Job drawing, mm, ordinate dimensions from the low corner. One solid piece. Round coordinates to 2 decimals unless told otherwise and drop trailing zeros. Order: outer loops, then holes, each group sorted by start corner. A loop starts at its lowest first (then second) coordinate and runs counter-clockwise, first axis right, second up. Notation, with made-up numbers: (15.25, 9.5) -> (57.25, 9.5) arc R20 ccw to (57.25, 48.5) -> close; hole circle Ø11 at (35, 71). An arc over 180 degrees is marked (long way). Use CSV: the item, a comma, the result in double quotes.
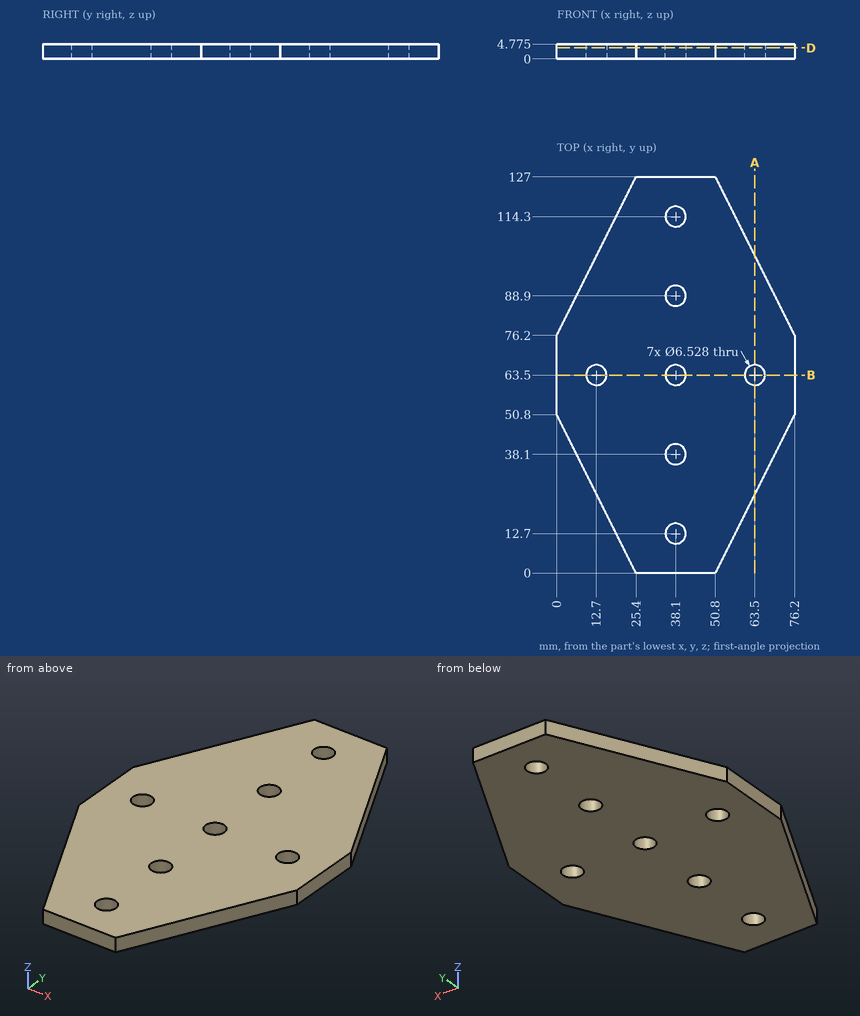
(1) Cut at B-B, the plane y = 63.5. Give the cut face in (x, z) (1 decimal).
Reply:
outline,"(0, 0) -> (9.4, 0) -> (9.4, 4.8) -> (0, 4.8) -> close; (16, 0) -> (34.8, 0) -> (34.8, 4.8) -> (16, 4.8) -> close; (41.4, 0) -> (60.2, 0) -> (60.2, 4.8) -> (41.4, 4.8) -> close; (66.8, 0) -> (76.2, 0) -> (76.2, 4.8) -> (66.8, 4.8) -> close"
(2) Probe probe 1 along Y at (x, z) = (38.1, 1.45); probe 2 along Y at (x, z) = (37.5, 0.6); probe 3 along Y at (x, z) = (63.5, 3.75) (1 decimal). List the from-to ranges inside material, lowest first. Write a range as [from, to].
Reply:
probe 1,"[0, 9.44], [15.96, 34.84], [41.36, 60.24], [66.76, 85.64], [92.16, 111.04], [117.56, 127]"
probe 2,"[0, 9.49], [15.91, 34.89], [41.31, 60.29], [66.71, 85.69], [92.11, 111.09], [117.51, 127]"
probe 3,"[25.4, 60.2], [66.8, 101.6]"
(3) Cut at D-D, the plane z = 3.5. Give the cut face in (x, y), then the cut area to 3 significant figures.
Reply:
outline,"(0, 50.8) -> (25.4, 0) -> (50.8, 0) -> (76.2, 50.8) -> (76.2, 76.2) -> (50.8, 127) -> (25.4, 127) -> (0, 76.2) -> close; hole circle Ø6.53 at (12.7, 63.5); hole circle Ø6.53 at (38.1, 12.7); hole circle Ø6.53 at (38.1, 38.1); hole circle Ø6.53 at (38.1, 63.5); hole circle Ø6.53 at (38.1, 88.9); hole circle Ø6.53 at (38.1, 114.3); hole circle Ø6.53 at (63.5, 63.5)"
area,"6,860 mm2"
(4) Cut at A-A, the plane x = 63.5. Give the cut face in (y, z) (1 decimal).
Reply:
outline,"(25.4, 0) -> (60.2, 0) -> (60.2, 4.8) -> (25.4, 4.8) -> close; (66.8, 0) -> (101.6, 0) -> (101.6, 4.8) -> (66.8, 4.8) -> close"
(5) Drop flat-ended pins along their axis: P1, Ø4, axis at x = 12.7, y = 63.5, coming from the -Z side; P2, Ø7.5, axis at x = 38.1, y = 114.3, coming from the +Z side (3 decimals); P3, Ø2, axis at y = 30, z = 1.5, coming from the -X side. Give the stop position or say it passes through.
Reply:
P1,"through"
P2,"z = 4.775"
P3,"x = 9.9"
